Part model, mm, in its own coordinate system. A direction names the side the tool comes from. Coordinates: 2 decimals unless noted, no trailing zeros. Write each loop counter-clockwise with the first axis right and the second up, starting at its lowest first coordinate (ties: lowest second). Pieces come first, ordered by that corner, then holes. Notation, with made-up numbers: M 79,87 L 138,87 A23 ccw 138,99 Z; hole C 16.25,-23 d6. An arc over 180 degrees is marked long. Use a Markdown table: item, result. Add a question column.
Q1. Wall check: L1, parallel to X at y = 11, z = -2.25 (3 decimals); L2, parallel to Y at x = -14, z = -2.5 (3 decimals); L3, parallel to Y at x = 0, z = -2.75. Give the ranges that are in metal, low to high. Write a range as from..to.
Q2. Tool access for faces 1 (the flat face through (20.32, 15, 1)), 2 (the cylindrical face through (-11.176, 15.708, -0.632)), 3 (the flat face through (-11.5, 11.535, -1.4)): list every direction of +Z, -Z, +X, -X, +Y, -Y with a clear straight run to the whole face (end or side of a thin tool).
Q3. Pin check, flat tips, straight feed: pin 1 Ø3 at (x, z) = (-12.7, 0) entering from +Y; pin 2 Ø1.6 at (x, z) = (12.5, -0.5) entering from -Y; pin 3 Ø1 at (x, y) = (9, 14) entering from -Z. Stop position of each tip, or through.
Q4. Slice it at D-D on x = 12. Write the cut outline in (y, z) (3 decimals), then the cut area to 3 significant figures.
Q5. Mould opens along X. For faces 4 (the flat face through (0, 13, -4.318)), 5 (the flat face through (8.74, 31.64, 0.94)), 6 (the cylindrical face through (14.224, 4.331, -0.632)) say: released by +X, released by -X, zero draft, split by the parting line, or undercut.
Q6. Slice it at C-C on y = 12. Write the cut outline in (x, z).
Autodesk Inventor part; units mm, degrees
ref_plane "Work Plane1" through (20.32, 0, -4.318) normal (0, 0, -1) x (-1, 0, 0)
ref_plane "Work Plane2" through (20.32, 0, -5.9055) normal (0, 0, -1) x (-1, 0, 0)
ref_plane "Work Plane3" through (0, 10.16, 0) normal (0, -1, 0) x (1, 0, 0)
sketch "Sketch3" plane through (0, 0, 0) normal (0, 1, 0) x (-1, 0, 0)
  line L0 (-20.32, 6.35) -> (20.32, 6.35)
  line L1 (20.32, 6.35) -> (20.32, -6.35)
  line L2 (20.32, -6.35) -> (-20.32, -6.35)
  line L3 (-20.32, -6.35) -> (-20.32, 6.35)
  line L4 (-20.32, 6.35) -> (20.32, -6.35) construction
  line L5 (20.32, 6.35) -> (-20.32, -6.35) construction
  point P0 (0, 0)
  dimension "d0" = 40.64
  dimension "d1" = 12.7
sketch "Sketch3 outline for Extrusion1" plane through (0, 0, 0) normal (0, 1, 0) x (-1, 0, 0)
  line L0 (-20.32, 6.35) -> (-20.32, -6.35)
  line L1 (20.32, 6.35) -> (-20.32, 6.35)
  line L2 (20.32, -6.35) -> (20.32, 6.35)
  line L3 (-20.32, -6.35) -> (20.32, -6.35)
extrude "Extrusion1" add sketch "Sketch3 outline for Extrusion1" along normal blind 30.48
sketch "Sketch4" plane through (-20.32, 0, 6.35) normal (0, 0, 1) x (1, 0, 0)
  line L0 (20.32, 0) -> (20.32, 24.13) construction
  circle A0 centre (20.32, 24.13) radius 4
  line L1 (12.7, 28.196818) -> (27.94, 28.196818)
  line L2 (27.94, 28.196818) -> (27.94, 32.763182)
  line L3 (27.94, 32.763182) -> (12.7, 32.763182)
  line L4 (12.7, 32.763182) -> (12.7, 28.196818)
  line L5 (40.64, 30.48) -> (0, 30.48)
  line L6 (12.7, 28.196818) -> (27.94, 32.763182) construction
  line L7 (27.94, 28.196818) -> (12.7, 32.763182) construction
  point P0 (20.32, 30.48)
  dimension "d4" = 24.13
  dimension "d5" = 8
  dimension "d6" = 15.24
sketch "Sketch4 outline for Extrusion2" plane through (-20.32, 0, 6.35) normal (0, 0, 1) x (1, 0, 0)
  line L0 (27.94, 32.763182) -> (12.7, 32.763182)
  line L1 (27.94, 28.196818) -> (27.94, 32.763182)
  line L2 (12.7, 28.196818) -> (27.94, 28.196818)
  line L3 (12.7, 32.763182) -> (12.7, 28.196818)
extrude "Extrusion2" add sketch "Sketch4 outline for Extrusion2" against normal up to surface (12.7 mm away)
sketch "Sketch4 outline for Extrusion3" plane through (-20.32, 0, 6.35) normal (0, 0, 1) x (1, 0, 0)
  circle A0 centre (20.32, 24.13) radius 4
extrude "Extrusion3" cut sketch "Sketch4 outline for Extrusion3" against normal blind 22.225
chamfer "Chamfer1" distance 2.28092 angle 45 2 edges at (7.62, 30.48, 0) (-7.62, 30.48, 0)
sketch "Sketch5" plane through (0, 0, 0) normal (0, -1, 0) x (1, 0, 0)
  line L0 (0, 0) -> (-12.7, 0) construction
  line L1 (0, 0) -> (12.7, 0) construction
  circle A0 centre (-12.7, 0) radius 1.65
  circle A1 centre (12.7, 0) radius 1.65
  dimension "d14" = 12.7
  dimension "d15" = 12.7
  dimension "d16" = 3.3
  dimension "d17" = 3.3
sketch "Sketch5 outline for Extrusion4" plane through (0, 0, 0) normal (0, -1, 0) x (1, 0, 0)
  circle A0 centre (12.7, 0) radius 1.65
  circle A1 centre (-12.7, 0) radius 1.65
extrude "Extrusion4" cut sketch "Sketch5 outline for Extrusion4" against normal blind 20
ref_plane "Work Plane1" through (20.32, 0, -4.318) normal (0, 0, -1) x (-1, 0, 0)
sketch "Sketch6" plane through (20.32, 0, -4.318) normal (0, 0, -1) x (-1, 0, 0)
  line L0 (0, 30.48) -> (10.41908, 30.48)
  line L1 (0, 0) -> (0, 30.48)
  line L2 (0, 0) -> (40.64, 0)
  line L3 (40.64, 0) -> (40.64, 30.48)
  line L4 (30.22092, 30.48) -> (40.64, 30.48)
  line L5 (27.94, 32.76092) -> (30.22092, 30.48)
  line L6 (12.7, 32.763182) -> (27.94, 32.763182)
  line L7 (10.41908, 30.48) -> (12.7, 32.76092)
  circle A0 centre (20.32, 24.13) radius 4
  line L8 (0, 30.48) -> (10.41908, 30.48)
  line L9 (0, 0) -> (0, 30.48)
  line L10 (0, 0) -> (40.64, 0)
  line L11 (40.64, 0) -> (40.64, 30.48)
  line L12 (30.22092, 30.48) -> (40.64, 30.48)
  line L13 (27.94, 32.76092) -> (30.22092, 30.48)
  line L14 (27.94, 32.763182) -> (27.94, 32.76092)
  line L15 (12.7, 32.763182) -> (27.94, 32.763182)
  line L16 (12.7, 32.76092) -> (12.7, 32.763182)
  line L17 (10.41908, 30.48) -> (12.7, 32.76092)
  line L18 (0, 30.48) -> (0, 0)
  line L19 (40.64, 0) -> (0, 0)
  line L20 (40.64, 0) -> (40.64, 30.48)
  line L21 (40.64, 30.48) -> (30.22092, 30.48)
  line L22 (30.22092, 30.48) -> (27.94, 32.763182)
  line L23 (27.94, 32.763182) -> (12.7, 32.76092)
  line L24 (12.7, 32.76092) -> (10.41908, 30.48)
  line L25 (0, 30.48) -> (10.41908, 30.48)
  point P0 (20.32, 0)
sketch "Sketch6 outline for Extrusion5" plane through (20.32, 0, -4.318) normal (0, 0, -1) x (-1, 0, 0)
  line L0 (27.94, 32.76092) -> (27.94, 32.763182)
  line L1 (30.22092, 30.48) -> (27.94, 32.76092)
  line L2 (27.94, 32.763182) -> (12.7, 32.76092)
  line L3 (40.64, 30.48) -> (30.22092, 30.48)
  line L4 (12.7, 32.76092) -> (10.41908, 30.48)
  line L5 (40.64, 0) -> (40.64, 30.48)
  line L6 (10.41908, 30.48) -> (0, 30.48)
  line L7 (0, 0) -> (40.64, 0)
  line L8 (0, 30.48) -> (0, 0)
  circle A0 centre (20.32, 24.13) radius 4
extrude "Extrusion5" cut sketch "Sketch6 outline for Extrusion5" along normal blind 20
sketch "Sketch7" plane through (20.32, 0, -4.318) normal (0, 0, -1) x (-1, 0, 0)
  circle A0 centre (20.32, 24.13) radius 8.255
  point P0 (20.32, 0)
ref_plane "Work Plane2" through (20.32, 0, -5.9055) normal (0, 0, -1) x (-1, 0, 0)
sketch "Sketch8" plane through (20.32, 0, -5.9055) normal (0, 0, -1) x (-1, 0, 0)
  circle A0 centre (20.32, 24.13) radius 5.5
  point P0 (20.32, 0)
  dimension "d25" = 11
sketch "Sketch7 outline for Loft1" plane through (20.32, 0, -4.318) normal (0, 0, -1) x (-1, 0, 0)
  circle A0 centre (20.32, 24.13) radius 8.255
sketch "Sketch8 outline for Loft1" plane through (20.32, 0, -5.9055) normal (0, 0, -1) x (-1, 0, 0)
  circle A0 centre (20.32, 24.13) radius 5.5
loft "Loft1" add profiles "Sketch7 outline for Loft1", "Sketch8 outline for Loft1"
sketch "Sketch9" plane through (-20.32, 0, 6.35) normal (0, 0, 1) x (1, 0, 0)
  circle A0 centre (20.32, 24.13) radius 4
  point P0 (20.32, 0)
sketch "Sketch9 outline for Extrusion6" plane through (-20.32, 0, 6.35) normal (0, 0, 1) x (1, 0, 0)
  circle A0 centre (20.32, 24.13) radius 4
extrude "Extrusion6" cut sketch "Sketch9 outline for Extrusion6" against normal blind 129.224999
ref_plane "Work Plane3" through (0, 10.16, 0) normal (0, -1, 0) x (1, 0, 0)
sketch "Sketch10" plane through (0, 10.16, 0) normal (0, -1, 0) x (1, 0, 0)
  circle A0 centre (-12.7, 0) radius 1.65
  line L0 (-15.5782, 0) -> (-9.87364, 0) construction
  line L1 (-9.90092, 1.631015) -> (-9.90092, -1.631015)
  line L2 (-15.55092, -1.631015) -> (-15.55092, 1.631015)
  line L3 (-12.72592, 3.262029) -> (-9.90092, 1.631015)
  line L4 (-15.55092, 1.631015) -> (-12.72592, 3.262029)
  line L5 (-12.72592, 0) -> (-9.90092, 0) construction
  line L6 (9.84772, 0) -> (15.55228, 0) construction
  line L7 (15.525, 1.631015) -> (15.525, -1.631015)
  line L8 (9.875, -1.631015) -> (9.875, 1.631015)
  line L9 (12.7, 3.262029) -> (15.525, 1.631015)
  line L10 (9.875, 1.631015) -> (12.7, 3.262029)
  line L11 (12.7, 0) -> (15.525, 0) construction
  circle A1 centre (12.7, 0) radius 1.65
  line L12 (15.525, -1.631015) -> (15.525, -3.262029)
  line L13 (15.525, -3.262029) -> (9.875, -3.262029)
  line L14 (9.875, -3.262029) -> (9.875, -1.631015)
  line L15 (-9.90092, -1.631015) -> (-9.90092, -3.262029)
  line L16 (-9.90092, -4.318) -> (-9.90092, 6.35)
  line L17 (-12.72592, -3.262029) -> (-9.90092, -3.262029)
  line L18 (-12.72592, -3.262029) -> (-15.55092, -3.262029)
  line L19 (-15.55092, -3.262029) -> (-15.55092, -1.631015)
  point P0 (0, 0)
  point P1 (-12.7, -1.132545)
  point P2 (-12.7, -3.5)
  point P3 (12.7, -1.132545)
  point P4 (12.7, -3.5)
  dimension "d34" = 2.825
  dimension "d35" = 2.825
sketch "Sketch10 outline for Extrusion7" plane through (0, 10.16, 0) normal (0, -1, 0) x (1, 0, 0)
  line L0 (-15.55092, -3.262029) -> (-9.90092, -3.262029)
  line L1 (-9.90092, -3.262029) -> (-9.90092, 1.631015)
  line L2 (-9.90092, 1.631015) -> (-12.72592, 3.262029)
  line L3 (-12.72592, 3.262029) -> (-15.55092, 1.631015)
  line L4 (-15.55092, 1.631015) -> (-15.55092, -3.262029)
  line L5 (15.525, 1.631015) -> (12.7, 3.262029)
  line L6 (12.7, 3.262029) -> (9.875, 1.631015)
  line L7 (9.875, 1.631015) -> (9.875, -3.262029)
  line L8 (9.875, -3.262029) -> (15.525, -3.262029)
  line L9 (15.525, -3.262029) -> (15.525, 1.631015)
extrude "Extrusion7" cut sketch "Sketch10 outline for Extrusion7" along normal mid plane 2.75
sketch "Sketch11" plane through (20.32, 0, -4.318) normal (0, 0, -1) x (-1, 0, 0)
  line L0 (29.08046, 32.526826) -> (11.260311, 32.526826)
  line L1 (11.260311, 32.526826) -> (11.260311, 35.082572)
  line L2 (11.260311, 35.082572) -> (29.08046, 35.082572)
  line L3 (29.08046, 35.082572) -> (29.08046, 32.526826)
  point P0 (20.32, 0)
sketch "Sketch11 outline for Extrusion8" plane through (20.32, 0, -4.318) normal (0, 0, -1) x (-1, 0, 0)
  line L0 (29.08046, 32.526826) -> (29.08046, 35.082572)
  line L1 (11.260311, 32.526826) -> (29.08046, 32.526826)
  line L2 (11.260311, 35.082572) -> (11.260311, 32.526826)
  line L3 (29.08046, 35.082572) -> (11.260311, 35.082572)
extrude "Extrusion8" cut sketch "Sketch11 outline for Extrusion8" along normal blind 9.949993
properties part number "Roller Bracket"
Recorded:
| question | item | result |
|---|---|---|
| 1 | L1 | -20.32..-15.551, -9.901..9.875, 15.525..20.32 |
| 1 | L2 | 0..8.785, 11.535..30.48 |
| 1 | L3 | 0..20.13, 28.13..32.76 |
| 2 | face 1 | +Z, -Z, +X, +Y, -Y |
| 2 | face 2 | -Y |
| 2 | face 3 | none |
| 3 | pin 1 | y = 30.48 |
| 3 | pin 2 | y = 20 |
| 3 | pin 3 | z = -4.32 |
| 4 | outline | M 0,-4.318 L 30.48,-4.318 L 30.48,6.35 L 0,6.35 L 0,1.494 L 8.785,1.494 L 8.785,2.858 L 11.535,2.858 L 11.535,1.494 L 20,1.494 L 20,-1.494 L 11.535,-1.494 L 11.535,-3.262 L 8.785,-3.262 L 8.785,-1.494 L 0,-1.494 Z |
| 4 | area | 257 mm² |
| 5 | face 4 | zero draft |
| 5 | face 5 | released by +X |
| 5 | face 6 | undercut |
| 6 | outline | M -20.32,-4.32 L 20.32,-4.32 L 20.32,6.35 L -20.32,6.35 Z; hole C -12.7,0 d3.3; hole C 12.7,0 d3.3 |
